Read the model definition and answer for the solid it produces. Units are mm, in the model's axes. A direction names the side the tool comes from. Coordinates: 2 decimals unless noted, no trailing zeros. Write each loop counter-clockwise with the first axis right and the second up, starting at its lowest first coordinate (ties: lowest second). Pieces come first, ordered by that corner, then holes. Notation, with made-up numbers: M -4.5,3 L 38.5,3 A13 cw 38.5,27 Z; hole C 61.5,4.25 d9. An arc over 180 degrees is marked long. Use a Markdown table: item, result. Add a question column.
from build123d import *

# Parameters (mm, degrees)
F0_R     = 11.811
F0_R_2   = 6.6675
F1_DEPTH = 64.77
F2_R     = 9.271
F2_R_2   = 6.6675
F2_R_3   = 11.811
F3_DEPTH = 11.049
F5_DEPTH = 3.429
F6_R     = 9.3345
F7_DEPTH = 9.398
F8_SIZE  = 1.5875


with BuildPart() as f1:
    # F0 (on Top) → F1 (new body)
    with BuildSketch(Plane.XY):
        Circle(F0_R)
        Circle(F0_R_2, mode=Mode.SUBTRACT)
    extrude(amount=F1_DEPTH)

    # F2 (on face) → F3 (cut)
    with BuildSketch(Plane(origin=(0, 0, 0), x_dir=(1, 0, 0), z_dir=(0, 0, -1))):
        Circle(F2_R)
        Circle(F2_R_2, mode=Mode.SUBTRACT)
        Circle(F2_R_3)
        Circle(F2_R, mode=Mode.SUBTRACT)
    extrude(amount=-F3_DEPTH, mode=Mode.SUBTRACT)

    # F4 (on face) → F5 (join)
    with BuildSketch(Plane(origin=(0, 0, 11.049), x_dir=(1, 0, 0), z_dir=(0, 0, -1))):
        with BuildLine():
            Line((1.7145, 11.176), (-1.7145, 11.176))
            Line((-1.7145, 11.176), (-1.7145, 9.111088))
            ThreePointArc((-1.7145, 9.111088), (0, 9.271), (1.7145, 9.111088))
            Line((1.7145, 9.111088), (1.7145, 11.176))
        make_face()
    extrude(amount=F5_DEPTH)

    # F6 (on face) → F7 (cut)
    with BuildSketch(Plane.XY.offset(64.77)):
        Circle(F6_R)
    extrude(amount=-F7_DEPTH, mode=Mode.SUBTRACT)

    # F8
    f8_edges = [f1.edges().sort_by_distance(p)[0] for p in [
        (-6.6675, 0, 55.372),
    ]]
    chamfer(f8_edges, length=F8_SIZE)


solid = f1.part
Item 1: Find section A-A on x = 0. Give the vertices of the cut face in (y, z) (1 decimal), then the cut area to 3 significant figures.
Item 2: Determine the mould class of faces 1 (the cylindrical face through (-2.01, 9.05, 5.45)), 2 (the cylindrical face through (-0.87, 6.61, 26.52)), 3 (the flat face through (3, -8, 55.372)), 4 (the flat face through (0, -10, 7.62)) for opening direction X: pulls with the +X half, pulls with the -X half, needs draft (parallel to the pull), parting line crosses it, or undercut.
Item 3: Each of these flat-tipped pins is pushed along its axis until it touches: pin 1 (1.7 mm diameter, centred on y = -10, z = 10, fed in from +X); pin 2 (6 mm diameter, centred on x = -8.5, z = 53.5, fed in from -Y); pin 3 (6 mm diameter, centred on y = 8, z = 12, fed in from -X); pin 4 (10.5 mm diameter, centred on x = 0, y = 0, fed in from +Z). Where does it stop, or does it pass through?
Item 4: Find section B-B on y = 0. Give the vertices of the cut face in (x, z) (1 decimal), then the cut area to 3 significant figures.
Item 5: Find section C-C on z = 42. Give the vertices of the cut face in (x, y) (1 decimal), then the cut area to 3 significant figures.
Item 6: For faces 5 (the flat face through (-1.714, -10, 9)), 6 (the cylindrical face through (8.903, 2.804, 60.137)), 7 (the flat face through (1.714, -10, 9)), 8 (the flat face through (0, -11.176, 9)), 9 (the cylindrical face through (-9.37, -7.19, 37.53)), determine the directions among +Z, -Z, +X, -X, +Y, -Y from which every point of the face is accessible in a straight line to the end or side of a thin tool.
Item 7: Consider probe 1 along X at (y, z) = (0, 27); probe 2 along Y at (x, z) = (0, 57.5); probe 3 along Y at (x, z) = (-0.25, 46.5). Determine where each line is inside the solid, lowest interval first.
Geometry says:
| question | item | result |
|---|---|---|
| 1 | outline | M -11.8,11 L -11.2,11 L -11.2,7.6 L -9.3,7.6 L -9.3,0 L -6.7,0 L -6.7,53.8 L -8.3,55.4 L -9.3,55.4 L -9.3,64.8 L -11.8,64.8 Z; M 6.7,0 L 9.3,0 L 9.3,11 L 11.8,11 L 11.8,64.8 L 9.3,64.8 L 9.3,55.4 L 8.3,55.4 L 6.7,53.8 Z |
| 1 | area | 564 mm2 |
| 2 | face 1 | parting line crosses it |
| 2 | face 2 | undercut |
| 2 | face 3 | undercut |
| 2 | face 4 | needs draft |
| 3 | pin 1 | stops at x = 1.71 |
| 3 | pin 2 | stops at y = -10.45 |
| 3 | pin 3 | stops at x = -10.7 |
| 3 | pin 4 | passes through |
| 4 | outline | M -11.8,11 L -9.3,11 L -9.3,0 L -6.7,0 L -6.7,53.8 L -8.3,55.4 L -9.3,55.4 L -9.3,64.8 L -11.8,64.8 Z; M 6.7,0 L 9.3,0 L 9.3,11 L 11.8,11 L 11.8,64.8 L 9.3,64.8 L 9.3,55.4 L 8.3,55.4 L 6.7,53.8 Z |
| 4 | area | 558 mm2 |
| 5 | outline | C 0,0 d23.6; hole C 0,0 d13.3 |
| 5 | area | 299 mm2 |
| 6 | face 5 | -Z, -X, -Y |
| 6 | face 6 | +Z |
| 6 | face 7 | -Z, +X, -Y |
| 6 | face 8 | -Z, +X, -X, -Y |
| 6 | face 9 | +Z, -Z |
| 7 | probe 1 | x = -11.81 to -6.67, 6.67 to 11.81 |
| 7 | probe 2 | y = -11.81 to -9.33, 9.33 to 11.81 |
| 7 | probe 3 | y = -11.81 to -6.66, 6.66 to 11.81 |
